Verification items for the finished model (mm, model axes). A direction names the side the tool comes from. Coordinates: 2 decimals unless noted, no trailing zeros. Order: outer loops, then holes, each group sorted by start corner. A loop starts at its lowest first (then second) coordinate and runs counter-clockwise, first axis right, second up. Notation, with made-up numbers: M -32.5,44.5 L -22.5,44.5 A14 cw -22.5,59.5 Z; hole C 50,38 d11. An arc over 180 degrees is marked long. Return JSON: item names as keys, results as strings.
```python
from build123d import *

# Parameters (mm, degrees)
SKETCH_1_R          = 1.5
EXTRUDE_1_DEPTH     = 3
CUT_EXTRUDE_1_DEPTH = 148.622791061
SKETCH_3_W          = 30
SKETCH_3_H          = 50
EXTRUDE_2_DEPTH     = 3
FILLET_1_R          = 3
SKETCH_4_R          = 2
CUT_EXTRUDE_2_DEPTH = 62.083894888
FILLET_2_R          = 5


with BuildPart() as part:
    # 草图1 → 凸台-拉伸1 (new body)
    with BuildSketch(Plane.XY):
        with BuildLine():
            ThreePointArc((74.735333077, -81.94640276), (73.202271099, -87.285997126), (78.48394402, -89.008053508))
            Line((78.48394402, -89.008053508), (92.427637923, -82.230635095))
            Line((92.427637923, -82.230635095), (117.427637923, -38.929364905))
            Line((117.427637923, -38.929364905), (116.32520749, -23.465062556))
            ThreePointArc((116.32520749, -23.465062556), (112.193026456, -19.752027824), (108.335333077, -23.749495625))
            Line((108.335333077, -23.749495625), (108.335333077, -32.677698856))
            Line((108.335333077, -32.677698856), (82.467383885, -77.482301144))
            Line((82.467383885, -77.482301144), (74.735333077, -81.94640276))
        make_face()
        with Locations((76.735333077, -85.410504375)):
            Circle(SKETCH_1_R, mode=Mode.SUBTRACT)
        with Locations((112.335333077, -23.749495625)):
            Circle(SKETCH_1_R, mode=Mode.SUBTRACT)
    extrude(amount=EXTRUDE_1_DEPTH)

    # 草图2 → 切除-拉伸1 (cut, through all)
    with BuildSketch(Plane.XY.offset(3)):
        with BuildLine():
            Line((93.432447394, -65.490254038), (103.432447394, -48.169745962))
            ThreePointArc((103.432447394, -48.169745962), (105.4814855, -47.620707856), (106.030523605, -49.669745962))
            Line((106.030523605, -49.669745962), (96.030523605, -66.990254038))
            ThreePointArc((96.030523605, -66.990254038), (93.9814855, -67.539292144), (93.432447394, -65.490254038))
        make_face()
    extrude(amount=-CUT_EXTRUDE_1_DEPTH, mode=Mode.SUBTRACT)

    # 草图3 → 凸台-拉伸2 (add)
    with BuildSketch(Plane(origin=(104.927637923, -60.58, 0), x_dir=(0, 0, -1), z_dir=(0.8660254037844419, -0.4999999999999942, 0))):
        with Locations((12, 0)):
            Rectangle(SKETCH_3_W, SKETCH_3_H)
    extrude(amount=EXTRUDE_2_DEPTH)

    # 圆角1
    fillet_1_edges = [part.edges().sort_by_distance(p)[0] for p in [
        (107.525714134, -62.08, 3),
        (104.927637923, -60.58, 0),
    ]]
    fillet(fillet_1_edges, radius=FILLET_1_R)

    # 草图4 → 切除-拉伸2 (cut, through all)
    with BuildSketch(Plane(origin=(107.525714134, -62.08, 0), x_dir=(0, 0, -1), z_dir=(0.8660254037844419, -0.4999999999999943, 0))):
        with BuildLine():
            Line((27, -25), (27, 25))
            Line((27, 25), (14, 25))
            ThreePointArc((14, 25), (17.5, 21.5), (14, 18))
            ThreePointArc((14, 18), (12.232233047, 17.267766953), (11.5, 15.5))
            Line((11.5, 15.5), (11.5, -15.5))
            ThreePointArc((11.5, -15.5), (12.232233047, -17.267766953), (14, -18))
            ThreePointArc((14, -18), (17.5, -21.5), (14, -25))
            Line((14, -25), (27, -25))
        make_face()
        with Locations(Location((5.5, 0, 0), (0, 0, 90))):
            Circle(SKETCH_4_R)
        with Locations(Location((5.5, 15, 0), (0, 0, 90))):
            Circle(SKETCH_4_R)
        with Locations(Location((5.5, -15, 0), (0, 0, 90))):
            Circle(SKETCH_4_R)
    extrude(amount=-CUT_EXTRUDE_2_DEPTH, mode=Mode.SUBTRACT)

    # 圆角2
    fillet_2_edges = [part.edges().sort_by_distance(p)[0] for p in [
        (82.467383885, -77.482301144, 1.5),
        (108.335333077, -32.677698856, 1.5),
    ]]
    fillet(fillet_2_edges, radius=FILLET_2_R)


solid = part.part
```
Q1. Material ranges on line 1 along Z through (x, y) = (81, -85); line 2 along X through (y, z) = (-64, -8.25); line 3 along Y through (x, z) = (116, -13.25), recorded low to high.
Values:
{"line 1": "0 to 3", "line 2": "102.95 to 106.42", "line 3": "-46.32 to -41.4"}
Q2. Go/stop test with flat-tipped pins: pin 1 (1.5 mm diameter, centred on y = -27.5, z = 1.5, fed in from -X); pin 2 (5 mm diameter, centred on y = -67, z = -12, fed in from +X); pin 3 (9 mm diameter, centred on x = 109.5, y = -61.5, fed in from -Z); pin 4 (3 mm diameter, centred on x = 94.5, y = -53.5, fed in from +Z). Record where each tip stops, or that it passes through.
Values:
{"pin 1": "x = 108.34", "pin 2": "x = 106.1", "pin 3": "z = -11.5", "pin 4": "through"}
Q3. Cross-section at D-D, the plane y = -30. Record the boundary of the cut face in (x, z).
Values:
{"outline": "M 108.34,0 L 116.79,0 L 116.79,3 L 108.34,3 Z"}
Q4. Cross-section at B-B, the plane z = -14.75. Record the boundary of the cut face in (x, y), and give its area (3 significant figures).
Values:
{"outline": "M 92.47,-82.16 L 95.07,-83.66 L 98.49,-77.74 L 95.89,-76.24 Z; M 113.97,-44.92 L 116.57,-46.42 L 119.99,-40.5 L 117.39,-39 Z", "area": "41.0 mm^2"}
Q5. Cross-section at A-A, the plane z = -4.5. Record the boundary of the cut face in (x, y), and give its area (3 significant figures).
Values:
{"outline": "M 92.43,-82.23 L 95.03,-83.73 L 99.16,-76.57 L 96.56,-75.07 Z; M 98.29,-72.07 L 100.89,-73.57 L 106.66,-63.58 L 104.06,-62.08 Z; M 105.79,-59.08 L 108.39,-60.58 L 114.16,-50.59 L 111.56,-49.09 Z; M 113.29,-46.09 L 115.89,-47.59 L 120.03,-40.43 L 117.43,-38.93 Z", "area": "119 mm^2"}
Q6. Cross-section at C-C, the plane z = -0.75. Record the boundary of the cut face in (x, y).
Values:
{"outline": "M 90.8,-83.02 L 92.43,-82.23 L 95.03,-83.73 L 120.03,-40.43 L 117.43,-38.93 L 117.3,-37.12 Z"}
Q7. Tool access check on faces 4 (the face through (98.362, -56.951, 1.521)), 5 (the face through (105.1, -60.28, -8.54)), 6 (the face through (93.71, -82.97, -5.38)). Record the directions out of +Z, -Z, +X, -X, +Y, -Y that give a thin tool (end or side, any length) a straight path to the whole face; none if there is none.
Values:
{"face 4": "+Z, -Z", "face 5": "-Z, -X, +Y", "face 6": "+Z, -Z, -Y"}
Q8. Draft check along Y on faces 1 (the face through (101.1, -58.21, 1.52)), 2 (the face through (106.92, -61.33, 2.14)), 3 (the face through (108.335, -27, 1)). Enter one of: pulls with the +Y half, pulls with the -Y half, needs draft (parallel to the pull), parting line crosses it, or undercut.
Values:
{"face 1": "undercut", "face 2": "pulls with the -Y half", "face 3": "needs draft"}
